```python
from build123d import *

# Parameters (mm, degrees)
BOSS_EXTRUDE1_DEPTH = 369.316
CUT_EXTRUDE1_DEPTH  = 17.526
CUT_EXTRUDE2_DEPTH  = 17.526


with BuildPart() as part:
    # Sketch1 → Boss-Extrude1 (new body)
    with BuildSketch(Plane(origin=(0, 0, 0), x_dir=(1, 0, 0), z_dir=(0, 1, 0))):
        Polygon((0, 38.1), (-6.35, 0), (-6.35, -5.08), (-3.175, -5.08), (-3.175, 0), (-1.5875, 0), (-1.5875, 2.54), (1.5875, 2.54), (1.5875, 0), (3.175, 0), (3.175, -5.08), (6.35, -5.08), (6.35, 0), align=None)
    extrude(amount=BOSS_EXTRUDE1_DEPTH)

    # Sketch2 → Cut-Extrude1 (cut)
    with BuildSketch(Plane.ZY.offset(6.35)):
        Polygon((5.08, 369.316), (-38.1, 294.223678497), (-38.1, 369.316), align=None)
    extrude(amount=-CUT_EXTRUDE1_DEPTH, mode=Mode.SUBTRACT)

    # Sketch3 → Cut-Extrude2 (cut)
    with BuildSketch(Plane.ZY.offset(6.35)):
        Polygon((5.08, 76.2), (-38.1, 1.107678497), (-38.1, 0), (5.08, 0), align=None)
    extrude(amount=-CUT_EXTRUDE2_DEPTH, mode=Mode.SUBTRACT)


solid = part.part
```
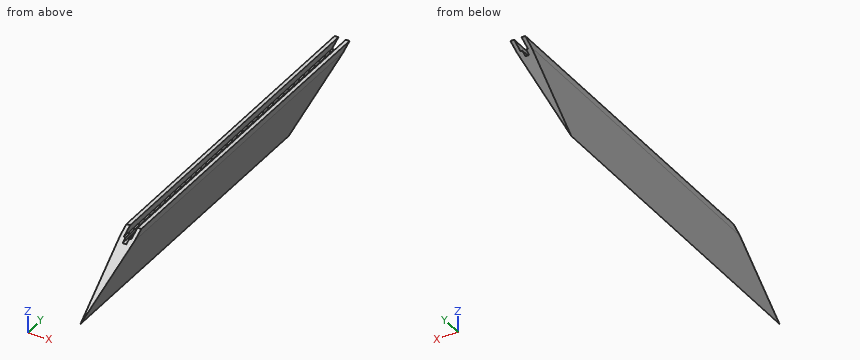
Source: CAD feature listing. Evaluate the final solid. Frame: model axes, mm. Coordinates: 2 decimals unless noted, no trailing zeros. Write each loop counter-clockwise with the first axis right and the second up, starting at its lowest first coordinate (ties: lowest second). Pieces come first, ordered by that corner, then holes. Notation, with made-up numbers: (-14, 75) -> (7, 75) arc R26 cw to (7, 106) -> close; hole circle Ø4 at (-11, 11). An arc over 180 degrees is marked (long way). Return JSON: item names as keys, results as strings. Group by question number.
1) Section query D-D, the plane y = 43. Return loops of the section in (x, z), plus the area to 3 significant figures.
2) Section query B-B, the plane z = -7.5. Return loops of the section in (x, y).
3) Section query C-C, the plane z = -34.5. Return loops of the section in (x, y).
4) Ray query, line 1 along X through (y, z) = (312.5, 3) (3 decimals); line 2 along X through (y, z) = (172.5, -2); line 3 along X through (y, z) = (304, -30.5). Return the intervals inside material, ascending.
5) Contact query for flat-ended pins moving along their axis: P1, Ø10, axis at y = 270.5, z = -28, coming from the +X side; P2, Ø8, axis at y = 52, z = -26.5, coming from the +X side; P3, Ø5, axis at x = -4, z = -1, coming from the -Y side; P4, Ø1.5, axis at x = 3, z = -33, coming from the +Y side. Output: stop coordinate, or through.
From the geometry:
{
 "1": {"outline": "(-4.01, -14.01) -> (0, -38.1) -> (4.01, -14.01) -> close", "area": "96.7 mm²"},
 "2": {"outline": "(-5.1, 54.32) -> (5.1, 54.32) -> (5.1, 347.44) -> (-5.1, 347.44) -> close"},
 "3": {"outline": "(-0.6, 7.37) -> (0.6, 7.37) -> (0.6, 300.48) -> (-0.6, 300.48) -> close"},
 "4": {"line 1": "-6.35 to -3.175, 3.175 to 6.35", "line 2": "-6.02 to -1.59, 1.59 to 6.02", "line 3": "-1.27 to 1.27"},
 "5": {"P1": "x = 2.52", "P2": "x = 2.6", "P3": "y = 61.28", "P4": "through"}
}
